Here's the drawing with two shaded views (mm, measured from the low corner). I have some questions. A direction names the side the tool comes from. Coordinates: 2 decimals unless noted, no trailing zeros. Write each loop counter-clockwise with the first axis right and the second up, starting at its lowest first coordinate (ties: lowest second). Pieces come first, ordered by that corner, then holes.
Item 1: We'd pull the mould along Z, two halves only. Please class the marked faces 1, 2, 3 and 4: +Z half, -Z half, draft (parallel to the pull), parting line (faces both ways), or undercut.
Item 2: I'm going to push flat-ended pins straight in: pin 1 Ø6 at (x, z) = (43.5, 5.3) entering from +Y; pin 2 Ø12.5 at (x, z) = (9, 27.5) entering from -Y; pin 3 Ø2.5 at (x, y) = (30, 3) entering from +Z; pin 4 Ø2.5 at (x, z) = (43.5, 20.6) entering from -Y. Where does each tip first touch, or does it pass through?
Item 3: If we section it at B-B (y = 6.25): Please give me the cut outline in (x, z).
Item 4: For the marked faces 5, 6 and 7, which set-ups out of +Z, -Z, +X, -X, +Y, -Y let a thin tool reach every point of the face, with its end or its side?
Item 5: If I drill on line 1 (Z direction, x = 9, y = 6.6); line 2 (Z direction, x = 44.5, y = 4.25) (1 decimal); line 3 (Z direction, x = 33, y = 3) (1 decimal), over which ranges is the centre line in solid material (lowest first)?
Item 6: If we section it at D-D (z = 9.5): Please give me the cut outline in (x, y).
Item 7: If we section it at A-A (x = 9): Please give me the cut outline in (y, z), then the cut area to 3 significant figures.
Item 8: If we section it at C-C (x = 43.5): Count the separate pieces of the cut face and the enclosed holes in it.
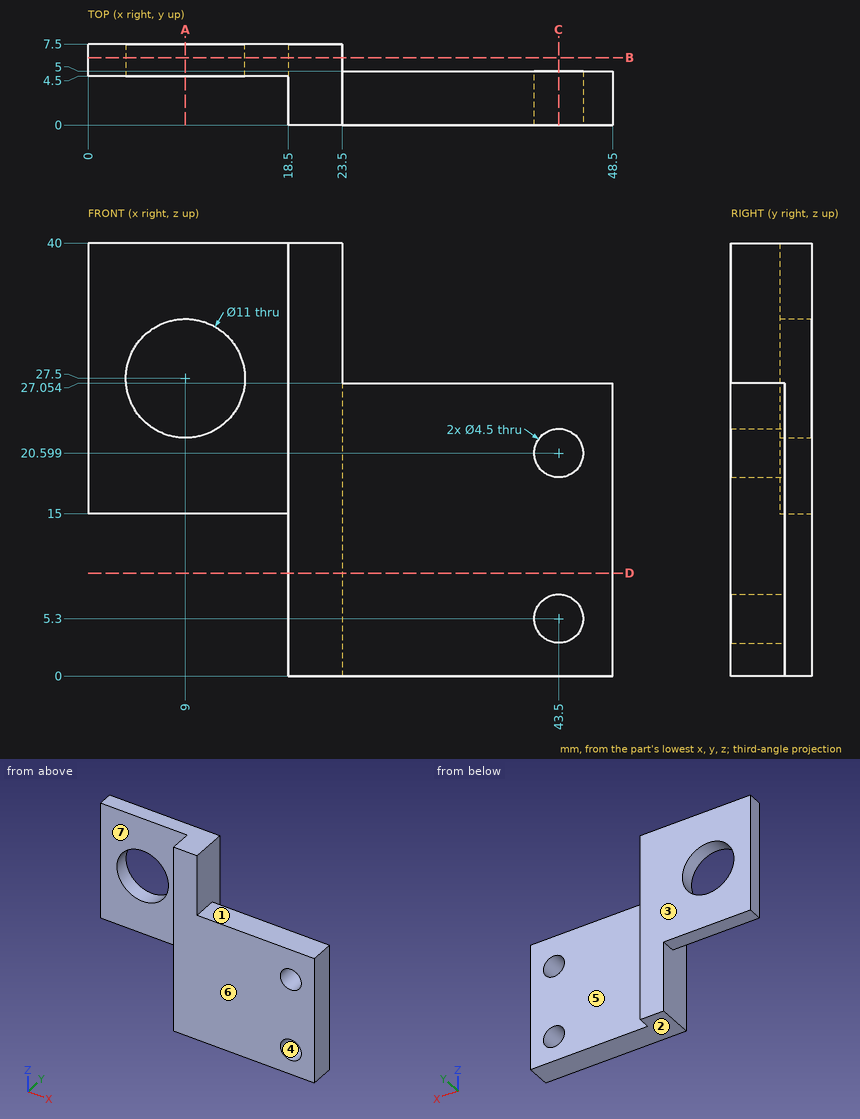
Answer list:
1. face 1: +Z half
1. face 2: -Z half
1. face 3: draft
1. face 4: undercut
2. pin 1: stops at y = 5
2. pin 2: stops at y = 4.5
2. pin 3: stops at z = 27.05
2. pin 4: passes through
3. outline: (0, 15) - (18.5, 15) - (18.5, 0) - (23.5, 0) - (23.5, 40) - (0, 40) - close; hole circle Ø11 at (9, 27.5)
4. face 5: +Z, -Z, +X, +Y
4. face 6: +Z, -Z, +X, -X, -Y
4. face 7: +Z, -Z, -X, -Y
5. line 1: z = 15 to 22, 33 to 40
5. line 2: z = 0 to 3.3, 7.3 to 18.6, 22.6 to 27.1
5. line 3: z = 0 to 27.1
6. outline: (18.5, 0) - (48.5, 0) - (48.5, 5) - (23.5, 5) - (23.5, 7.5) - (18.5, 7.5) - close
7. outline: (4.5, 15) - (7.5, 15) - (7.5, 22) - (4.5, 22) - close; (4.5, 33) - (7.5, 33) - (7.5, 40) - (4.5, 40) - close
7. area: 42.0 mm2
8. separate pieces: 3
8. enclosed holes: 0
